Geometry: final body of the model. Coordinates: model frame, mm. A direction names the side the tool comes from. Coordinates: 2 decimals unless noted, no trailing zeros. Order: outer loops, then holes, each group sorted by start corner. A loop starts at its lowest first (then second) coordinate and runs counter-clockwise, first axis right, second up. Notation, with made-up numbers: (61, 46) -> (94, 46) arc R25 cw to (94, 67) -> close; hole circle Ø8 at (6.25, 72.5). An arc over 180 degrees is marked (long way). Answer in a Markdown table with one row per item. Add a question column.
1) Pull-direction query (Y, two-part tool) for faces 4 (the face through (16.69, 44.74, -3.92)), 5 (the face through (18, 50.4, -5)), 6 (the face through (0, 30, -9.85)); classes: +Y half, -Y half, draft (parallel to the pull), parting line (faces both ways), or undercut.
2) Section query C-C on z = 0.5. Return the cut outline in (x, y), then the cut area to 3 significant figures.
3) Section query A-A on y = 15.7. Return the cut outline in (x, z), then the cut area to 3 significant figures.
4) Section query D-D on y = 56. Return the cut outline in (x, z).
5) Contact query for flat-ended pins moving along their axis: P1, Ø4.5, axis at x = 0.5, y = 29.5, coming from the +Z side; P2, Ø7, axis at x = 20, z = 2, coming from the +Y side; P3, Ø2.5, axis at x = -19.5, z = -1.5, coming from the -Y side. Output: stop coordinate, or through.
6) Ray query, line 1 (Y direction, x = -19, z = -1); line 2 (X direction, y = 5, z = 2.5); line 3 (Y direction, x = 20.5, z = -6). Return the intervals inside material, ascending. Write a range as from..to.
7) Section query B-B on z = -5. Return the cut outline in (x, y).
8) Set-up query: faces 1 (the face through (-18, 50.4, -5)), 2 (the face through (21, 31, -0.95)), 3 (the face through (15.041, 56, 0)). Return all of +Z, -Z, +X, -X, +Y, -Y with unobstructed straight access to the full face (end or side cutting, diameter ignored); none if empty.
```python
from build123d import *

# Parameters (mm, degrees)
SKETCH_5_W          = 47
SKETCH_5_H          = 19.7
EXTRUDE_3_DEPTH     = 61.4
CUT_EXTRUDE_1_DEPTH = 62.4
CUT_EXTRUDE_2_DEPTH = 11
SKETCH_8_R          = 2.5
CUT_EXTRUDE_3_DEPTH = 33
SKETCH_9_W          = 15
SKETCH_9_H          = 21.981640809
CUT_EXTRUDE_4_DEPTH = 73


with BuildPart() as part:
    # 草图5 → 凸台-拉伸3 (new body)
    with BuildSketch(Plane(origin=(0, 0, 0), x_dir=(1, 0, 0), z_dir=(0, 1, 0))):
        Rectangle(SKETCH_5_W, SKETCH_5_H)
    extrude(amount=EXTRUDE_3_DEPTH)

    # 草图6 → 切除-拉伸1 (cut, through all)
    with BuildSketch(Plane(origin=(0, 61.4, 0), x_dir=(1, 0, 0), z_dir=(0, 1, 0))):
        Polygon((-18.819510237, 0.95), (-23.5, 0.95), (-23.5, -9.85), (-15.040666545, -9.85), align=None)
        Polygon((18.819510237, 0.95), (15.040666545, -9.85), (23.5, -9.85), (23.5, 0.95), align=None)
    extrude(amount=-CUT_EXTRUDE_1_DEPTH, mode=Mode.SUBTRACT)

    # 草图6<6> → 切除-拉伸2 (cut)
    with BuildSketch(Plane(origin=(0, 61.4, 0), x_dir=(1, 0, 0), z_dir=(0, 1, 0))):
        Polygon((-19, 9.85), (-23.5, 9.85), (-23.5, 0.95), (-18.819510237, 0.95), (-15.040666545, -9.85), (-15.040666545, 9.85), align=None)
        Polygon((19, 9.85), (15.040666545, 9.85), (15.040666545, -9.85), (18.819510237, 0.95), (23.5, 0.95), (23.5, 9.85), align=None)
    cut_extrude_2 = extrude(amount=-CUT_EXTRUDE_2_DEPTH, mode=Mode.SUBTRACT)

    # 镜向1: 切除-拉伸2 across plane
    add(cut_extrude_2.mirror(Plane.ZX.offset(30.7)), mode=Mode.SUBTRACT)

    # 草图8 → 切除-拉伸3 (cut)
    with BuildSketch(Plane(origin=(0, 0, -9.85), x_dir=(-1, 0, 0), z_dir=(0, 0, -1))):
        with Locations((-19, 15.7)):
            Circle(SKETCH_8_R)
        with Locations((19, 15.7)):
            Circle(SKETCH_8_R)
        with Locations((19, 45.7)):
            Circle(SKETCH_8_R)
        with Locations((-19, 45.7)):
            Circle(SKETCH_8_R)
    extrude(amount=-CUT_EXTRUDE_3_DEPTH, mode=Mode.SUBTRACT)

    # 草图9 → 切除-拉伸4 (cut)
    with BuildSketch(Plane.XZ):
        with Locations((0, 10.140820404)):
            Rectangle(SKETCH_9_W, SKETCH_9_H)
    extrude(amount=-CUT_EXTRUDE_4_DEPTH, mode=Mode.SUBTRACT)


solid = part.part
```
Result:
| question | item | result |
|---|---|---|
| 1 | face 4 | undercut |
| 1 | face 5 | +Y half |
| 1 | face 6 | draft |
| 2 | outline | (-18.31, 11) -> (-15.04, 11) -> (-15.04, 0) -> (-7.5, 0) -> (-7.5, 61.4) -> (-15.04, 61.4) -> (-15.04, 50.4) -> (-18.31, 50.4) -> (-18.31, 48.1) arc R2.5 cw to (-18.31, 43.3) -> (-18.31, 18.1) arc R2.5 cw to (-18.31, 13.3) -> close; (7.5, 0) -> (15.04, 0) -> (15.04, 11) -> (18.31, 11) -> (18.31, 13.3) arc R2.5 cw to (18.31, 18.1) -> (18.31, 43.3) arc R2.5 cw to (18.31, 48.1) -> (18.31, 50.4) -> (15.04, 50.4) -> (15.04, 61.4) -> (7.5, 61.4) -> close |
| 2 | area | 1,160 mm2 |
| 3 | outline | (-23.5, -9.85) -> (-21.5, -9.85) -> (-21.5, -0.95) -> (-23.5, -0.95) -> close; (-16.5, -9.85) -> (16.5, -9.85) -> (16.5, 5.68) -> (15.04, 9.85) -> (7.5, 9.85) -> (7.5, -0.85) -> (-7.5, -0.85) -> (-7.5, 9.85) -> (-15.04, 9.85) -> (-16.5, 5.68) -> close; (21.5, -9.85) -> (23.5, -9.85) -> (23.5, -0.95) -> (21.5, -0.95) -> close |
| 3 | area | 519 mm2 |
| 4 | outline | (-15.04, -9.85) -> (15.04, -9.85) -> (15.04, 9.85) -> (7.5, 9.85) -> (7.5, -0.85) -> (-7.5, -0.85) -> (-7.5, 9.85) -> (-15.04, 9.85) -> close |
| 5 | P1 | z = -0.85 |
| 5 | P2 | y = 50.4 |
| 5 | P3 | y = 11 |
| 6 | line 1 | 11..13.2, 18.2..43.2, 48.2..50.4 |
| 6 | line 2 | -15.04..-7.5, 7.5..15.04 |
| 6 | line 3 | 11..13.7, 17.7..43.7, 47.7..50.4 |
| 7 | outline | (-23.5, 11) -> (-15.04, 11) -> (-15.04, 0) -> (15.04, 0) -> (15.04, 11) -> (23.5, 11) -> (23.5, 50.4) -> (15.04, 50.4) -> (15.04, 61.4) -> (-15.04, 61.4) -> (-15.04, 50.4) -> (-23.5, 50.4) -> close; hole circle Ø5 at (-19, 15.7); hole circle Ø5 at (-19, 45.7); hole circle Ø5 at (19, 15.7); hole circle Ø5 at (19, 45.7) |
| 8 | face 1 | +Z, -Z, -X, +Y |
| 8 | face 2 | +Z, +X, +Y, -Y |
| 8 | face 3 | +Z, -Z, +X, +Y |
